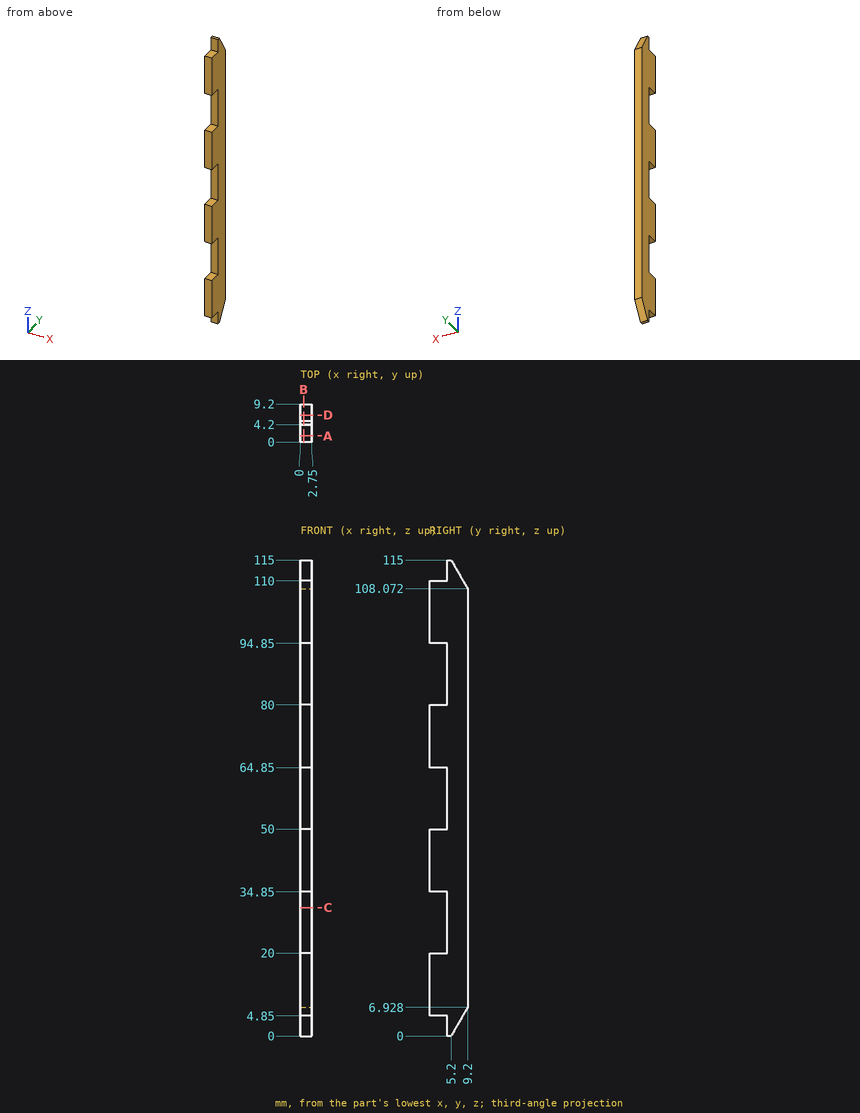
Job drawing, mm, ordinate dimensions from the low corner. One solid piece. Give positions to 0.01 mm unless a question says otherwise; leave off trailing zeros. Order: outer loops, then holes, each group sorted by start corner. A loop starts at its lowest first (then second) coordinate and runs counter-clockwise, first axis right, second up. Notation, with made-up numbers: M 56,45 L 80,45 A9 cw 80,55 Z; hole C -30.75,17.5 d7. An arc over 180 degrees is marked long. Put each result on its own line as item: value. Start each with the question number.
(1) Pin check, flat tips, straight feed: pin 1 Ø1.4 at (x, y) = (1, 2) entering from +Z; pin 2 Ø1.4 at (x, y) = (2, 3) entering from -Z; pin 3 Ø1 at (x, y) = (0.5, 7.5) entering from -Z. Stop position of each tip, or through.
(2) Band-saw the part on A-A on y = 1.5. Give the cut face in (x, z).
(3) Band-saw the part on C-C on z = 31. Give the cut face in (x, y).
(4) Band-saw the part on B-B on x = 0.8. Give the cut face in (y, z), then the cut area to 3 significant figures.
(5) Drill centre lines: L1, parallel to Z at x = 1.55, y = 1.5; L2, parallel to Y at x = 1.45, z = 90; L3, parallel to Z at x = 1.3, y = 5.25 (1 decimal). Where is each one in solid material? Low to high. Write a range as [from, to].
(6) Band-saw the part on D-D on y = 6.5. Give the cut face in (x, z).
Results below:
1. pin 1: stops at z = 110
1. pin 2: stops at z = 4.85
1. pin 3: stops at z = 3.12
2. outline: M 0,4.85 L 2.75,4.85 L 2.75,20 L 0,20 Z; M 0,34.85 L 2.75,34.85 L 2.75,50 L 0,50 Z; M 0,64.85 L 2.75,64.85 L 2.75,80 L 0,80 Z; M 0,94.85 L 2.75,94.85 L 2.75,110 L 0,110 Z
3. outline: M 0,4.2 L 2.75,4.2 L 2.75,9.2 L 0,9.2 Z
4. outline: M 0,4.85 L 4.2,4.85 L 4.2,0 L 5.2,0 L 9.2,6.93 L 9.2,108.07 L 5.2,115 L 4.2,115 L 4.2,110 L 0,110 L 0,94.85 L 4.2,94.85 L 4.2,80 L 0,80 L 0,64.85 L 4.2,64.85 L 4.2,50 L 0,50 L 0,34.85 L 4.2,34.85 L 4.2,20 L 0,20 Z
4. area: 802 mm2
5. L1: z = [4.85, 20], [34.85, 50], [64.85, 80], [94.85, 110]
5. L2: y = [4.2, 9.2]
5. L3: z = [0.1, 114.9]
6. outline: M 0,2.25 L 2.75,2.25 L 2.75,112.75 L 0,112.75 Z
